Design review of the part built by this model. Coordinates are the model's own, in mm. A direction names the side the tool comes from. Coordinates: 2 decimals unless noted, no trailing zeros. Write each loop counter-clockwise with the first axis right and the second up, starting at its lowest first coordinate (ties: lowest second). Pieces come first, ordered by that corner, then holes.
Q1. Add section D-D, the plane z = 25. Give the boundary of the cut face in (x, y).
Q2. Add section A-A, the plane y = 0. Give the boundary of the cut face in (x, z).
Q3. To check wall thickness, follow probe 1 along X at (y, z) = (16, 0); probe 2 along X at (y, z) = (-28, -4); probe 3 along Z at (x, y) = (-2.5, -2). State the ranges of each line that lie inside material, in increasing order.
Q4. Machinability: for faces 1 (the face through (-200, 0, 0)), 2 (the face through (240, -30.4, 8.5)), which of the approach directions +Z, -Z, +X, -X, +Y, -Y give a long, thin tool a straight path to every point of the face, cutting with its end or side? Answer none if there is none.
Q5. Add section B-B, the plane z = 0. Give the boundary of the cut face in (x, y), plus the area to 3 significant figures.
Q6. Add section C-C, the plane x = 290. Give the boundary of the cut face in (y, z).
Q7. Clearance check with flat-ended pins moving along their axes: pin 1 Ø17.5 at (x, z) = (-150, 0) entering from +Y; pin 2 Ø8 at (x, y) = (-129, -25) entering from -Z; pin 3 Ø3 at (x, z) = (81, 22) entering from +Y; pin 4 Ø1 at (x, y) = (41, -22) entering from -Z. State where each tip first meets the part, or that it passes through.
Q8. The part is to be moulded in two halves that separate along X. For faces 3 (the face through (-101.4, -9.414, -29.893)), 4 (the face through (379.26, -0.44, -2.38)), 5 (the face through (0, -30.4, 8.5)), say which applies: +X half, -X half, draft (parallel to the pull), parting line (faces both ways), or undercut.
from build123d import *

# Parameters (mm, degrees)
SKETCH1_R               = 37.5
BOSS_EXTRUDE1_DEPTH     = 240
SKETCH2_R               = 31.34
BOSS_EXTRUDE2_DEPTH     = 200
BOSS_EXTRUDE3_START     = 200
SKETCH3_R               = 31.34
BOSS_EXTRUDE3_DEPTH     = 200
CUT_EXTRUDE1_DEPTH      = 444.184498826
CUT_EXTRUDE1_DEPTH_BACK = 444.184498826
SKETCH4_R               = 11


with BuildPart() as part:
    # Sketch1 → Boss-Extrude1 (new body)
    with BuildSketch(Plane(origin=(0, 0, 0), x_dir=(0, 0, -1), z_dir=(1, 0, 0))):
        Circle(SKETCH1_R)
    extrude(amount=BOSS_EXTRUDE1_DEPTH)

    # Sketch2 → Boss-Extrude2 (add)
    with BuildSketch(Plane(origin=(240, 0, 0), x_dir=(0, 0, -1), z_dir=(1, 0, 0))):
        Circle(SKETCH2_R)
    extrude(amount=BOSS_EXTRUDE2_DEPTH)

    # Sketch3 → Boss-Extrude3 (add)
    with BuildSketch(Plane.ZY.offset(BOSS_EXTRUDE3_START)):
        with Locations(Location((0, 0, 0), (0, 0, 180))):
            Circle(SKETCH3_R)
    extrude(amount=-BOSS_EXTRUDE3_DEPTH)

    # Sketch4 → Cut-Extrude1 (cut, two sides: drawn at the far end of the back side and taken through both)
    with BuildSketch(Plane(origin=(0, 0, 0), x_dir=(1, 0, 0), z_dir=(0, 1, 0)).offset(-CUT_EXTRUDE1_DEPTH_BACK)):
        with Locations(Location((-50, 0, 0), (0, 0, 270))):
            Circle(SKETCH4_R)
        with Locations(Location((-150, 0, 0), (0, 0, 270))):
            Circle(SKETCH4_R)
        with Locations(Location((290, 0, 0), (0, 0, 270))):
            Circle(SKETCH4_R)
        with Locations(Location((390, 0, 0), (0, 0, 270))):
            Circle(SKETCH4_R)
    extrude(amount=CUT_EXTRUDE1_DEPTH + CUT_EXTRUDE1_DEPTH_BACK, mode=Mode.SUBTRACT)


solid = part.part
Here are the results:
1. outline: (-200, -18.9) - (0, -18.9) - (0, -27.95) - (240, -27.95) - (240, -18.9) - (440, -18.9) - (440, 18.9) - (240, 18.9) - (240, 27.95) - (0, 27.95) - (0, 18.9) - (-200, 18.9) - close
2. outline: (-200, -31.34) - (0, -31.34) - (0, -37.5) - (240, -37.5) - (240, -31.34) - (440, -31.34) - (440, 31.34) - (240, 31.34) - (240, 37.5) - (0, 37.5) - (0, 31.34) - (-200, 31.34) - close; hole circle Ø22 at (-150, 0); hole circle Ø22 at (-50, 0); hole circle Ø22 at (290, 0); hole circle Ø22 at (390, 0)
3. probe 1: x = -200 to -161, -139 to -61, -39 to 279, 301 to 379, 401 to 440
3. probe 2: x = -200 to -160.25, -139.75 to -60.25, -39.75 to 279.75, 300.25 to 379.75, 400.25 to 440
3. probe 3: z = -31.28 to 31.28
4. face 1: +Z, -Z, -X, +Y, -Y
4. face 2: +X
5. outline: (-200, -31.34) - (-161, -31.34) - (-161, 31.34) - (-200, 31.34) - close; (-139, -31.34) - (-61, -31.34) - (-61, 31.34) - (-139, 31.34) - close; (-39, -31.34) - (0, -31.34) - (0, -37.5) - (240, -37.5) - (240, -31.34) - (279, -31.34) - (279, 31.34) - (240, 31.34) - (240, 37.5) - (0, 37.5) - (0, 31.34) - (-39, 31.34) - close; (301, -31.34) - (379, -31.34) - (379, 31.34) - (301, 31.34) - close; (401, -31.34) - (440, -31.34) - (440, 31.34) - (401, 31.34) - close
5. area: 37,600 mm2
6. outline: (-29.35, -11) arc R31.34 ccw to (29.35, -11) - close; (-29.35, 11) - (29.35, 11) arc R31.34 ccw to start
7. pin 1: passes through
7. pin 2: stops at z = -23.26
7. pin 3: stops at y = 31.4
7. pin 4: stops at z = -30.72
8. face 3: draft
8. face 4: undercut
8. face 5: -X half
